Input: part model. Units: mm. Frame: model coordinates. Round coordinates to 2 decimals unless told otherwise and drop trailing zeros. Order: outer loops, then holes, each group sorted by start corner. A loop starts at its lowest first (then second) coordinate and runs counter-clockwise, first axis right, second up. Notation, with made-up numbers: M 75,57.5 L 99,57.5 A31 ccw 99,81.5 Z; hole C 64.25,10.5 d3. An arc over 180 degrees is marked long. One line per question, with ' | ' between items.
```python
from build123d import *

# Parameters (mm, degrees)
ESQUISSE1_W          = 36
ESQUISSE1_H          = 26
BOSS_EXTRU_1_DEPTH   = 8
D_GAGEMENT_M41_D     = 4.5
M6_CLEARANCE_HOLE2_D = 6.6


with BuildPart() as part:
    # Esquisse1 → Boss.-Extru.1 (new body)
    with BuildSketch(Plane.XY):
        Rectangle(ESQUISSE1_W, ESQUISSE1_H)
    extrude(amount=BOSS_EXTRU_1_DEPTH)

    # Dégagement M41 (through all)
    with Locations(Plane(origin=(0, 0, 0), x_dir=(-1, 0, 0), z_dir=(0, 0, -1))):
        with Locations((-11.318887596, -0.107841378), (10.681112224, -0.10502754)):
            Hole(D_GAGEMENT_M41_D / 2)

    # M6 Clearance Hole2 (through all)
    with Locations(Plane(origin=(0, 0, 0), x_dir=(-1, 0, 0), z_dir=(0, 0, -1))):
        with Locations((-2.073526459, 0)):
            Hole(M6_CLEARANCE_HOLE2_D / 2)


solid = part.part
```
Item 1: First-contact query: pin 1 (7 mm diameter, centred on x = -10.68, y = -0.11, fed in from -Z). Flat tip, straight axial feed; report the tip coordinate or a pass-through.
Report:
pin 1: z = 0
Item 2: Section query C-C, the plane x = 10. Return loops of the section in (y, z), plus the area to 3 significant figures.
Report:
outline: M -13,0 L -1.93,0 L -1.93,8 L -13,8 Z; M 1.72,0 L 13,0 L 13,8 L 1.72,8 Z | area: 179 mm²
Item 3: Section query B-B, the plane z = 3.75. Return loops of the section in (x, y).
Report:
outline: M -18,-13 L 18,-13 L 18,13 L -18,13 Z; hole C -10.68,-0.11 d4.5; hole C 2.07,0 d6.6; hole C 11.32,-0.11 d4.5
Item 4: Line query: line 1 along X through (y, z) = (1, 7.75); line 2 along X through (y, z) = (-2, 1.75); line 3 along Y through (x, z) = (3.5, 5). Output: solid intervals per line, ascending. Write a range as from..to.
Report:
line 1: -18..-12.64, -8.72..-1.07, 5.22..9.36, 13.28..18 | line 2: -18..-11.89, -9.47..-0.55, 4.7..10.1, 12.54..18 | line 3: -13..-2.98, 2.98..13
Item 5: Mould query, pull axis X, two halves, no side actions, for faces 1 (the flat face through (-18, 0, 4)), 2 (the cylindrical face through (10.831, -2.304, 4.056)), 3 (the flat face through (18, 0, 4)), 4 (the flat face through (0, -13, 4)). Classes: +X half, -X half, draft (parallel to the pull), parting line (faces both ways), or undercut.
Report:
face 1: -X half | face 2: undercut | face 3: +X half | face 4: draft
Item 6: Section query A-A, the plane x = -0.5. Return loops of the section in (y, z), plus the area to 3 significant figures.
Report:
outline: M -13,0 L -2.07,0 L -2.07,8 L -13,8 Z; M 2.07,0 L 13,0 L 13,8 L 2.07,8 Z | area: 175 mm²
